CAD build for the part. Positions are in the model's coordinates, mm. A direction names the side the tool comes from. Give positions to 0.01 mm unless a question says otherwise; leave off trailing zeros. Write each loop counter-clockwise with the first axis right and the second up, starting at its lowest first coordinate (ties: lowest second). Pieces come first, ordered by that corner, then holes. Notation, with made-up numbers: (7, 89.25) -> (48, 89.25) arc R18 ccw to (48, 114.25) -> close; hole circle Ø6 at (40.5, -35.75). An arc over 180 degrees is marked (long way). Answer as a JSON object with one key per item and string values.
```python
from build123d import *

# Parameters (mm, degrees)
CYLINDER023_R     = 13
CYLINDER023_DEPTH = 23
CYLINDER024_R     = 15.5
CYLINDER024_DEPTH = 23
CYLINDER025_R     = 13
CYLINDER025_DEPTH = 40
BOX001_W          = 23
BOX001_H          = 31
BOX001_DEPTH      = 20
SKETCH005_R       = 0.5
PAD004_DEPTH      = 3


with BuildPart() as cylinder023:
    # Cylinder023 → Cylinder023 (new body)
    with BuildSketch(Plane(origin=(0, 0, 7), x_dir=(0, 0, -1), z_dir=(1, 0, 0))):
        Circle(CYLINDER023_R)
    extrude(amount=CYLINDER023_DEPTH)


with BuildPart() as cut:
    # Cylinder024 → Cylinder024 (new body)
    with BuildSketch(Plane(origin=(0, 0, 7), x_dir=(0, 0, -1), z_dir=(1, 0, 0))):
        Circle(CYLINDER024_R)
    extrude(amount=CYLINDER024_DEPTH)

    # Cut: cut Cylinder023
    add(cylinder023.part, mode=Mode.SUBTRACT)


with BuildPart() as cut_1:
    # Cut placement: moved
    add(cut.part.moved(Location((-11.5, 0, 13.5))))


with BuildPart() as cylinder025:
    # Cylinder025 → Cylinder025 (new body)
    with BuildSketch(Plane(origin=(-17, 0, 20.5), x_dir=(0, 0, -1), z_dir=(1, 0, 0))):
        Circle(CYLINDER025_R)
    extrude(amount=CYLINDER025_DEPTH)


with BuildPart() as cut001:
    # Box001 → Box001 (new body)
    with BuildSketch(Plane(origin=(-11.5, -15.5, 0), x_dir=(1, 0, 0), z_dir=(0, 0, 1))):
        with Locations((11.5, 15.5)):
            Rectangle(BOX001_W, BOX001_H)
    extrude(amount=BOX001_DEPTH)

    # Cut001: cut Cylinder025
    add(cylinder025.part, mode=Mode.SUBTRACT)


with BuildPart() as obj1:
    # Sketch005 → Pad004 (new body)
    with BuildSketch(Plane.XY):
        with BuildLine():
            Line((-13.625988, 19), (14.385989, 19))
            ThreePointArc((19, 14.385989), (17.648587, 17.648587), (14.385989, 19))
            Line((19, 14.385989), (19, -14.278508))
            ThreePointArc((14.278508, -19), (17.617107, -17.617107), (19, -14.278508))
            Line((14.278508, -19), (-14.385989, -19))
            ThreePointArc((-19, -14.385989), (-17.648587, -17.648587), (-14.385989, -19))
            Line((-19, -14.385989), (-19, 13.625988))
            ThreePointArc((-13.625988, 19), (-17.425988, 17.425988), (-19, 13.625988))
        make_face()
        with Locations((-14, 14)):
            Circle(SKETCH005_R, mode=Mode.SUBTRACT)
        with Locations((14, 14)):
            Circle(SKETCH005_R, mode=Mode.SUBTRACT)
        with Locations((14, -14)):
            Circle(SKETCH005_R, mode=Mode.SUBTRACT)
        with Locations((-14, -14)):
            Circle(SKETCH005_R, mode=Mode.SUBTRACT)
    extrude(amount=PAD004_DEPTH)

    # Fusion027: union Cut, Cut001
    add(cut_1.part)
    add(cut001.part)


solid = obj1.part
```
1) Slice it at A-A (y = 0). List the corners of the cut face in (x, z), then the cut area to 3 significant figures.
Model answer:
{"outline": "(-19, 0) -> (19, 0) -> (19, 3) -> (11.5, 3) -> (11.5, 7.5) -> (-11.5, 7.5) -> (-11.5, 3) -> (-19, 3) -> close; (-11.5, 33.5) -> (11.5, 33.5) -> (11.5, 36) -> (-11.5, 36) -> close", "area": "275 mm2"}
2) 3-axis set-ups, long thin cutter, end or side, ignore diameter. For faces 4 (the flat face through (11.5, -7, 8)), 5 (the flat face through (0, -15.5, 11)), 6 (the flat face through (0, 15.5, 11)): which of +Z, -Z, +X, -X, +Y, -Y reach the whole face in a straight line?
Model answer:
{"face 4": "+Z, +X, +Y, -Y", "face 5": "+Z, +X, -X, -Y", "face 6": "+Z, +X, -X, +Y"}
3) Slice it at C-C (z = 32). List the corners of the cut face in (x, y).
Model answer:
{"outline": "(-11.5, -10.39) -> (11.5, -10.39) -> (11.5, -6.06) -> (-11.5, -6.06) -> close; (-11.5, 6.06) -> (11.5, 6.06) -> (11.5, 10.39) -> (-11.5, 10.39) -> close"}
4) Mould opens along X. For faces 1 (the cylindrical face through (17.58, -17.654, 1.479)), 2 (the cylindrical face through (-0.2, 3.9, 8.1)), 3 (the cylindrical face through (13.935, -13.504, 1.479)) say: released by +X, released by -X, zero draft, split by the parting line, or undercut.
Model answer:
{"face 1": "released by +X", "face 2": "zero draft", "face 3": "undercut"}
5) Slice it at D-D (z = 26). List the corners of the cut face in (x, y), then the cut area to 3 significant figures.
Model answer:
{"outline": "(-11.5, -14.49) -> (11.5, -14.49) -> (11.5, -11.78) -> (-11.5, -11.78) -> close; (-11.5, 11.78) -> (11.5, 11.78) -> (11.5, 14.49) -> (-11.5, 14.49) -> close", "area": "125 mm2"}
6) Wall check: probe 1 along Y at (x, z) = (14, 2.15); probe 2 along Z at (x, y) = (6, 0); probe 3 along Y at (x, z) = (-5.25, 20.5). Give the ranges that are in metal, low to high.
Model answer:
{"probe 1": "y = -19 to -14.5, -13.5 to 13.5, 14.5 to 19", "probe 2": "z = 0 to 7.5, 33.5 to 36", "probe 3": "y = -15.5 to -13, 13 to 15.5"}
7) Pin check, flat tips, straight feed: pin 1 (12 mm diameter, centred on y = 4, z = 11, fed in from +X); pin 2 (8.5 mm diameter, centred on x = -2, z = 7.5, fed in from +Y); pin 3 (5 mm diameter, centred on y = -14, z = 30, fed in from -X); pin 4 (9.5 mm diameter, centred on y = 2, z = 15.5, fed in from -X). Stop position of each tip, or through.
Model answer:
{"pin 1": "stops at x = 11.5", "pin 2": "stops at y = 15.5", "pin 3": "stops at x = -11.5", "pin 4": "passes through"}
